Answer from the drawing. Dimensions are ordinates in mm from the lowest x, y and z of the part. A direction names the side the tool comes from. Give positions to 0.01 mm unless a question says otherwise; leave off trailing zeros. Loops run counter-clockwise (first coordinate to the right, second up) from the corner with the lowest first, then second, coordinate; pieces in that order, holes last.
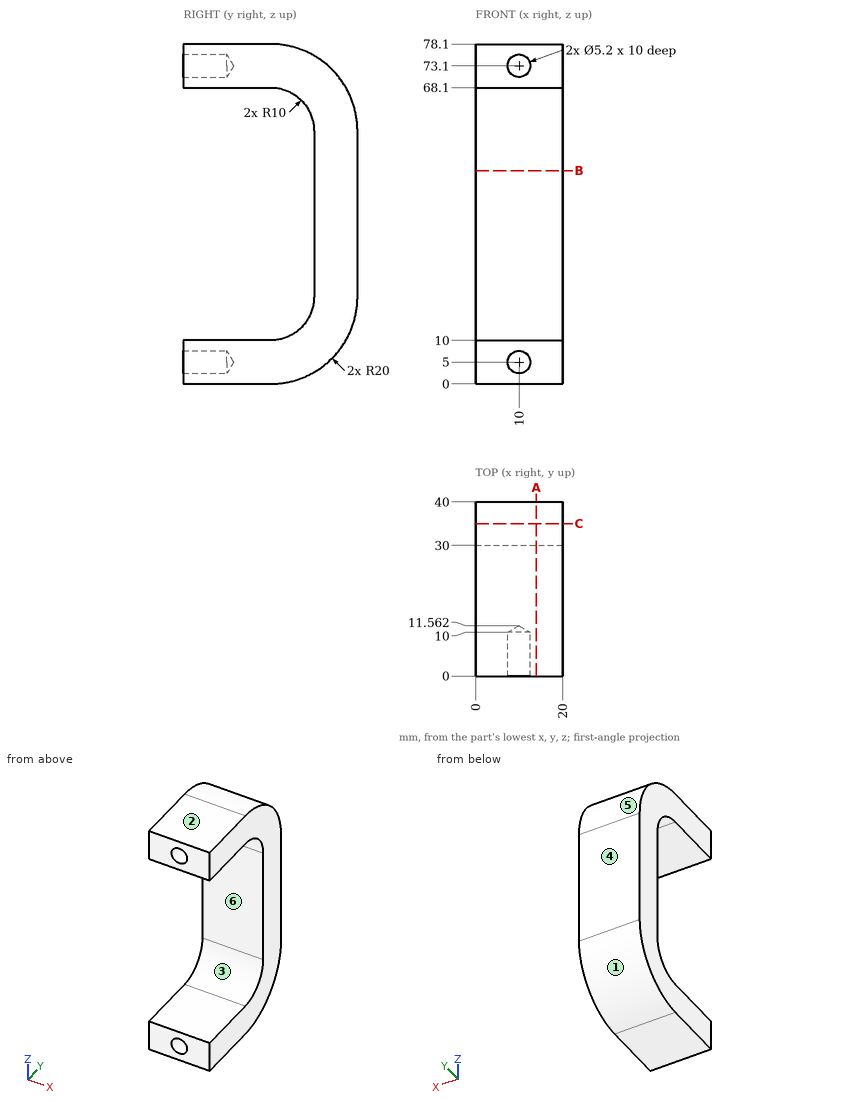
Item 1: Flat-ended cylindrical pins translate along their axes: pin 1 Ø5 at (x, z) = (10.5, 20.5) entering from -Y; pin 2 Ø1.5 at (x, z) = (6.5, 31.5) entering from -Y; pin 3 Ø3 at (x, y) = (16.5, 18.5) entering from -Z; pin 4 Ø4 at (x, z) = (10, 73.1) entering from +Y. Find the tip coordinate at first contact, or state that the pin passes through.
Item 2: Determine the mould class of the marked faces 1, 2, 3 and 4 for opening direction Z: released by +Z, released by -Z, zero draft, split by the parting line, or undercut.
Item 3: Consider line 1 (Z direction, x = 10, y = 7.5); line 2 (X direction, y = 3, z = 5); line 3 (Z direction, x = 18, y = 19). Determine where each line is inside the solid, lowest interval first.
Item 4: Find section B-B, the plane z = 49. Write down the section's boundary in (x, y), plus the area to 3 significant figures.
Item 5: For the marked faces 5 and 6, determine the directions among +Z, -Z, +X, -X, +Y, -Y from which every point of the face is accessible in a straight line to the end or side of a thin tool.
Item 6: Find section A-A, the plane x = 14. Write down the section's boundary in (y, z).
Item 7: Find section C-C, the plane y = 35. Write down the section's boundary in (x, z).
Ans:
1. pin 1: stops at y = 29.8
1. pin 2: stops at y = 30
1. pin 3: stops at z = 0
1. pin 4: stops at y = 35.2
2. face 1: released by -Z
2. face 2: released by +Z
2. face 3: undercut
2. face 4: zero draft
3. line 1: z = 0 to 2.4, 7.6 to 10, 68.1 to 70.5, 75.7 to 78.1
3. line 2: x = 0 to 7.4, 12.6 to 20
3. line 3: z = 0 to 10, 68.1 to 78.1
4. outline: (0, 30) - (20, 30) - (20, 40) - (0, 40) - close
4. area: 200 mm2
5. face 5: +Z, +X, -X, +Y
5. face 6: +X, -X, -Y
6. outline: (0, 0) - (20, 0) arc R20 ccw to (40, 20) - (40, 58.1) arc R20 ccw to (20, 78.1) - (0, 78.1) - (0, 68.1) - (20, 68.1) arc R10 cw to (30, 58.1) - (30, 20) arc R10 cw to (20, 10) - (0, 10) - close
7. outline: (0, 6.77) - (20, 6.77) - (20, 71.33) - (0, 71.33) - close
